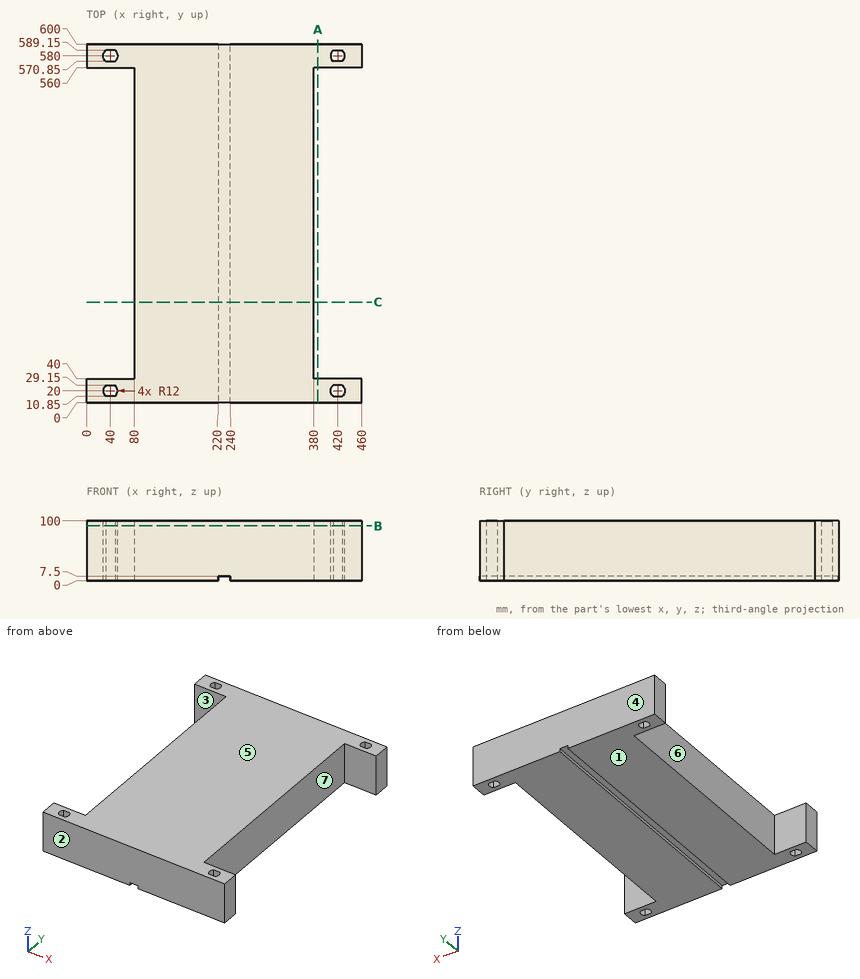
Source: three-view drawing plus pictorial views. Frame: mm from the lowest corner of the part. A direction names the side the tool comes from. Give positions to 0.01 mm unless a question says otherwise; leave off trailing zeros. Loops run counter-clockwise (first coordinate to the right, second up) from the corner with the lowest first, then second, coordinate; pieces in that order, holes last. Notation, with made-up numbers: (1.5, 29) -> (40.5, 29) arc R28 cw to (40.5, 47) -> close; hole circle Ø6 at (84.5, 28.25). An arc over 180 degrees is marked (long way). Put each result on its own line as item: value. Start each with the question number.
1) Cut plane B-B (z = 91.5). Return loops of the section in (x, y).
2) Contact query for flat-ended pins moving along their axis: P1, Ø10, axis at y = 128.5, z = 61.5, coming from the -X side; P2, Ø8, axis at y = 311, z = 2.5, coming from the +X side. Output: stop coordinate, or through.
3) Material intervals for probe 1 along Y at (x, z) = (33, 5.5); probe 2 along Y at (x, z) = (21, 36.5); probe 3 along X at (y, z) = (386, 33), sorted ascending.
4) Cut plane A-A (x = 387). Return loops of the section in (y, z), then the cut area to 3 significant figures.
5) Cut plane C-C (y = 168.5). Return loops of the section in (x, z), then the cut area to 4 significant figures.
6) Reachability of the marked faces 5, 6 and 7 from +Z, -Z, +X, -X, +Y, -Y: full face, straight path, thin tool, end or side. Return the list, or none.
7) Draft query along Y for the marked faces 1, 2, 3 and 4. Return one class per face: released by +Y, released by -Y, zero draft, split by the parting line, or undercut.
Results are:
1. outline: (0, 0) -> (460, 0) -> (460, 40) -> (380, 40) -> (380, 560) -> (460, 560) -> (460, 600) -> (0, 600) -> (0, 560) -> (80, 560) -> (80, 40) -> (0, 40) -> close; hole (32.24, 10.85) -> (47.76, 10.85) arc R12 ccw to (47.76, 29.15) -> (32.24, 29.15) arc R12 ccw to start; hole (32.24, 570.85) -> (47.76, 570.85) arc R12 ccw to (47.76, 589.15) -> (32.24, 589.15) arc R12 ccw to start; hole (412.24, 10.85) -> (427.76, 10.85) arc R12 ccw to (427.76, 29.15) -> (412.24, 29.15) arc R12 ccw to start; hole (412.24, 570.85) -> (427.76, 570.85) arc R12 ccw to (427.76, 589.15) -> (412.24, 589.15) arc R12 ccw to start
2. P1: stops at x = 80
2. P2: stops at x = 380
3. probe 1: y = 0 to 10.85, 29.15 to 40, 560 to 570.85, 589.15 to 600
3. probe 2: y = 0 to 40, 560 to 600
3. probe 3: x = 80 to 380
4. outline: (0, 0) -> (40, 0) -> (40, 100) -> (0, 100) -> close; (560, 0) -> (600, 0) -> (600, 100) -> (560, 100) -> close
4. area: 8,000 mm2
5. outline: (80, 0) -> (220, 0) -> (220, 7.5) -> (240, 7.5) -> (240, 0) -> (380, 0) -> (380, 100) -> (80, 100) -> close
5. area: 29,850 mm2
6. face 5: +Z, +X, -X, +Y, -Y
6. face 6: +Z, -Z, -X
6. face 7: +Z, -Z, +X
7. face 1: zero draft
7. face 2: released by -Y
7. face 3: undercut
7. face 4: released by +Y
